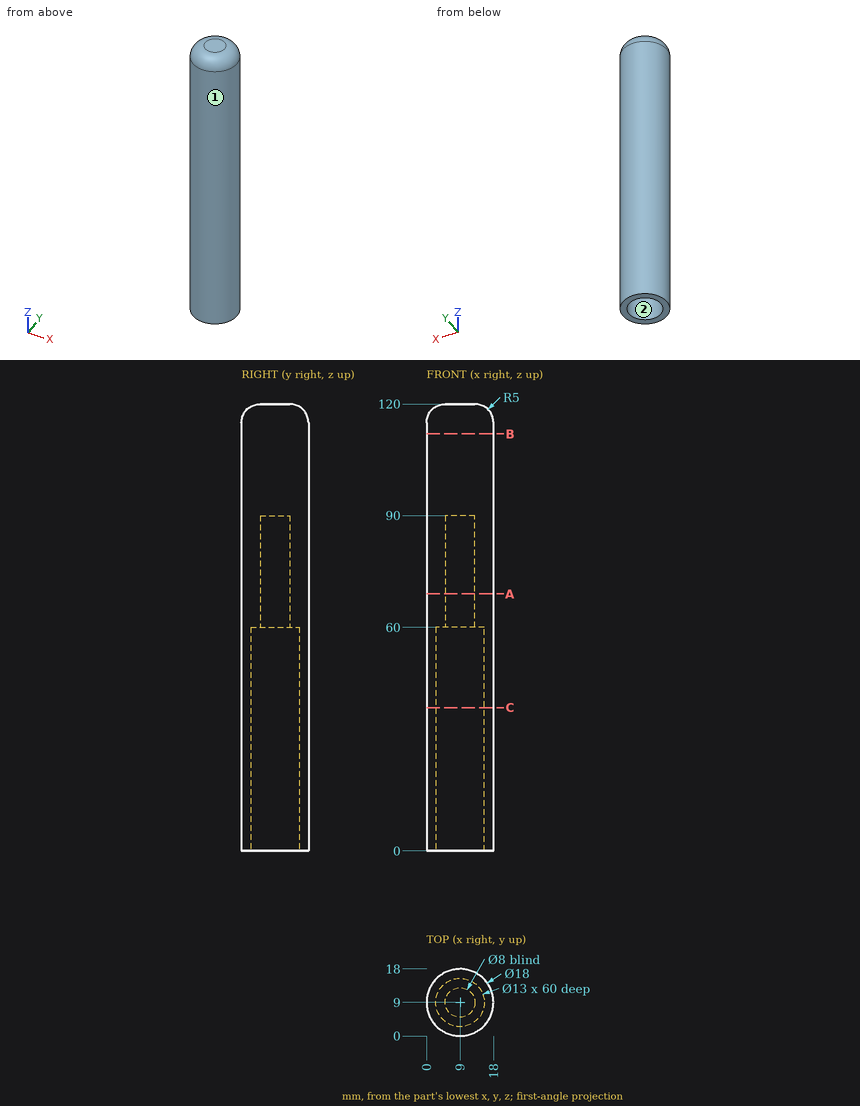
Could you check a few things on this drawing? It's one solid part, dimensions in mm from its lowest x, y, z. Coordinates: 2 decimals unless noted, no trailing zeros. Write each loop counter-clockwise with the first axis right and the second up, starting at its lowest first coordinate (ties: lowest second). Pieces come first, ordered by that corner, then holes. Notation, with made-up numbers: (-26.75, 18) - (7.25, 18) arc R15 ccw to (7.25, 35) - close; hole circle Ø7 at (5.5, 50.25). An arc over 180 degrees is marked (long way). Return JSON: item names as keys, results as strings. Group by question number.
Item 1: If we section it at C-C (z = 38.5): Write out the boundary of the cut face in (x, y), then the cut area to 3 significant figures.
Item 2: Please list where these lines run through material, in increasing order: probe 1 along Y at (x, z) = (9, 29); probe 2 along Y at (x, z) = (9, 68.5); probe 3 along X at (y, z) = (13, 24.5).
Item 3: I'm going to push flat-ended pins straight in: pin 1 Ø1.5 at (x, z) = (12.5, 37) entering from -Y; pin 2 Ø1.5 at (y, z) = (7, 73.5) entering from -X; pin 3 Ø6 at (y, z) = (15, 76) entering from +X. Where does each tip first touch, or does it pass through?
Item 4: If we section it at B-B (z = 112): Write out the boundary of the cut face in (x, y), then the cut area to 3 significant figures.
Item 5: We'd pull the mould along X, two halves only. Please class the marked faces 1 and 2: pulls with the +X half, pulls with the -X half, needs draft (parallel to the pull), parting line crosses it, or undercut.
Item 6: If we section it at A-A (z = 69): Write out the boundary of the cut face in (x, y), then the cut area to 3 significant figures.
Return value:
{
 "1": {"outline": "circle Ø18 at (9, 9); hole circle Ø13 at (9, 9)", "area": "122 mm^2"},
 "2": {"probe 1": "y = 0 to 2.5, 15.5 to 18", "probe 2": "y = 0 to 5, 13 to 18", "probe 3": "x = 0.94 to 3.88, 14.12 to 17.06"},
 "3": {"pin 1": "stops at y = 0.43", "pin 2": "stops at x = 0.09", "pin 3": "stops at x = 17.49"},
 "4": {"outline": "circle Ø18 at (9, 9)", "area": "254 mm^2"},
 "5": {"face 1": "parting line crosses it", "face 2": "undercut"},
 "6": {"outline": "circle Ø18 at (9, 9); hole circle Ø8 at (9, 9)", "area": "204 mm^2"}
}
